from build123d import *

# Parameters (mm, degrees)
F1_DEPTH = 13.081
F2_R     = 2.54
F3_DEPTH = 25.4
F4_R     = 3.4925
F5_DEPTH = 25.4
F6_SIZE2 = 1.4664696837
F6_SIZE  = 2.54
F7_R     = 5.08


with BuildPart() as f1:
    # F0 (on Top) → F1 (new body)
    with BuildSketch(Plane.XY):
        with BuildLine():
            ThreePointArc((3.1717183454, 34.7806818182), (21.0354315126, 27.8794950829), (32.574512842, 12.5959016393))
            ThreePointArc((32.574512842, 12.5959016393), (33.9739390049, 10.8274361777), (36.1280960611, 10.16))
            Line((36.1280960611, 10.16), (40.005, 10.16))
            ThreePointArc((40.005, 10.16), (41.8010512242, 9.4160512242), (42.545, 7.62))
            Line((42.545, 7.62), (42.545, -7.62))
            Line((42.545, -7.62), (55.245, -7.62))
            Line((55.245, -7.62), (55.245, 5.1702561211))
            ThreePointArc((55.245, 5.1702561211), (54.9549810189, 6.6282799984), (54.1290768363, 7.8643329574))
            Line((54.1290768363, 7.8643329574), (21.8343329574, 40.1590768363))
            ThreePointArc((21.8343329574, 40.1590768363), (20.5982799984, 40.9849810189), (19.1402561211, 41.275))
            Line((19.1402561211, 41.275), (0, 41.275))
            Line((0, 41.275), (-56.515, 41.275))
            Line((-56.515, 41.275), (-56.515, 18.415))
            Line((-56.515, 18.415), (-43.815, 18.415))
            ThreePointArc((-43.815, 18.415), (-42.0189487758, 17.6710512242), (-41.275, 15.875))
            Line((-41.275, 15.875), (-41.275, 0))
            ThreePointArc((-41.275, 0), (-40.8262821798, -6.0696217652), (-39.4898851183, -12.0072727273))
            ThreePointArc((-39.4898851183, -12.0072727273), (-37.9470586927, -13.8847124809), (-35.528565284, -14.1213198343))
            ThreePointArc((-35.528565284, -14.1213198343), (-34.7738270947, -13.7787585984), (-34.1334673575, -13.252529236))
            ThreePointArc((-34.1334673575, -13.252529236), (-33.3596724116, -11.8025855442), (-33.414518177, -10.16))
            ThreePointArc((-33.414518177, -10.16), (-33.8417993799, -8.6306569699), (-34.1991233561, -7.0834727836))
            ThreePointArc((-34.1991233561, -7.0834727836), (-33.8811086179, 8.4750282492), (-26.836399518, 22.3509124179))
            ThreePointArc((-26.836399518, 22.3509124179), (-24.6957043329, 24.6957043329), (-22.3509124179, 26.836399518))
            ThreePointArc((-22.3509124179, 26.836399518), (-13.3652188754, 32.266492673), (-3.1717183454, 34.7806818182))
            ThreePointArc((-3.1717183454, 34.7806818182), (0, 34.925), (3.1717183454, 34.7806818182))
        make_face()
        with BuildLine():
            ThreePointArc((-26.836399518, 22.3509124179), (-22.4506403027, 22.4506403027), (-22.3509124179, 26.836399518))
            ThreePointArc((-22.3509124179, 26.836399518), (-24.6957043329, 24.6957043329), (-26.836399518, 22.3509124179))
        make_face()
        with BuildLine():
            ThreePointArc((-32.3537599551, -13.1525602742), (-30.3768347063, -9.2363636364), (-34.1991233561, -7.0834727836))
            ThreePointArc((-34.1991233561, -7.0834727836), (-33.8417993799, -8.6306569699), (-33.414518177, -10.16))
            ThreePointArc((-33.414518177, -10.16), (-32.9181630162, -11.6683404405), (-32.3537599551, -13.1525602742))
        make_face()
        with BuildLine():
            ThreePointArc((-32.3537599551, -13.1525602742), (-32.9181630162, -11.6683404405), (-33.414518177, -10.16))
            ThreePointArc((-33.414518177, -10.16), (-33.3596724116, -11.8025855442), (-34.1334673575, -13.252529236))
            ThreePointArc((-34.1334673575, -13.252529236), (-33.3085642944, -13.333231598), (-32.4908818133, -13.1976834706))
            ThreePointArc((-32.4908818133, -13.1976834706), (-32.422064403, -13.175901276), (-32.3537599551, -13.1525602742))
        make_face()
        with BuildLine():
            ThreePointArc((-32.4908818133, -13.1976834706), (-33.3085642944, -13.333231598), (-34.1334673575, -13.252529236))
            ThreePointArc((-34.1334673575, -13.252529236), (-34.7738270947, -13.7787585984), (-35.528565284, -14.1213198343))
            Line((-35.528565284, -14.1213198343), (-32.4908818133, -13.1976834706))
        make_face()
        with BuildLine():
            ThreePointArc((-3.1717183454, 34.7806818182), (0, 31.75), (3.1717183454, 34.7806818182))
            ThreePointArc((3.1717183454, 34.7806818182), (0, 34.925), (-3.1717183454, 34.7806818182))
        make_face()
    extrude(amount=F1_DEPTH)

    # F2 (on face) → F3 (cut)
    with BuildSketch(Plane.YZ.offset(55.245)):
        with Locations((-1.2248719395, 6.5405)):
            Circle(F2_R)
    extrude(amount=-F3_DEPTH, mode=Mode.SUBTRACT)

    # F4 (on face) → F5 (cut)
    with BuildSketch(Plane(origin=(0, 41.275, 0), x_dir=(-1, 0, 0), z_dir=(0, 1, 0))):
        with Locations((48.895, 6.5405)):
            Circle(F4_R)
    extrude(amount=-F5_DEPTH, mode=Mode.SUBTRACT)

    # F6
    f6_edges = [f1.edges().sort_by_distance(p)[0] for p in [
        (-45.4025, 41.275, 6.5405),
        (-45.4025, 18.415, 6.5405),
    ]]
    f6_side = f1.faces().sort_by_distance((-45.4025, 29.845, 6.5405))[0]
    chamfer(f6_edges, length=F6_SIZE, length2=F6_SIZE2, reference=f6_side)

    # F7
    f7_edges = [f1.edges().sort_by_distance(p)[0] for p in [
        (-56.515, 29.845, 13.081),
        (-56.515, 29.845, 0),
        (48.895, -7.62, 13.081),
        (48.895, -7.62, 0),
    ]]
    fillet(f7_edges, radius=F7_R)


solid = f1.part
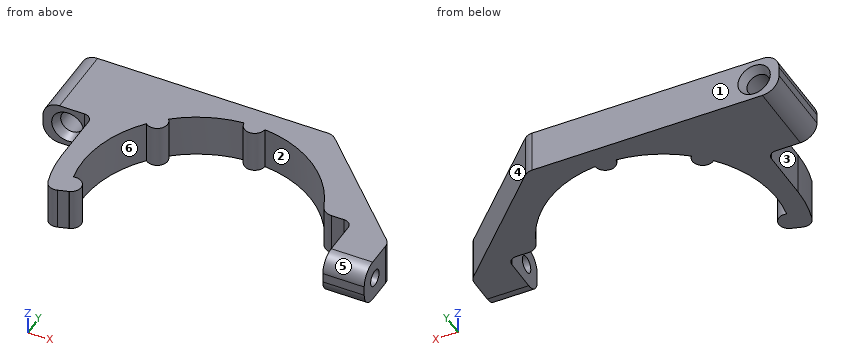
Design review of the part built by this model. Coordinates are the model's own, in mm. Face numbers are marked on the shaded views. A direction names the side the tool comes from. Coordinates: 2 decimals unless noted, no trailing zeros. Order: outer loops, then holes, each group sorted by start corner. A loop starts at its lowest first (then second) coordinate and runs counter-clockwise, first axis right, second up.
Item 1: Take a section at A-A, the plane y = 24. Write out the cut boundary in (x, z) (1 decimal).
Item 2: Take a section at B-B, the plane y = 17. Write out the cut boundary in (x, z).
Item 3: Take a section at D-D, the plane y = -10.16. Write out the cut boundary in (x, z) (3 decimals), then the cut area to 3 significant figures.
Item 4: For line 1 (Y direction, x = 48.5, z = 8.75); line 2 (X direction, y = 28, z = 8) (3 decimals); line 3 (Y direction, x = -30.5, z = 8.25) (3 decimals), list the stretches that pass through material, from the lowest coordinate up.
Item 5: The part is to be moulded in two halves that separate along X. For the marked faces 4, 5 and 6, say which applies: pulls with the +X half, pulls with the -X half, needs draft (parallel to the pull), parting line crosses it, or undercut.
Item 6: For pin 1 Ø2 at (y, z) = (6.5, 3) entering from -X (3 decimals); pin 2 Ø4.5 at (y, z) = (-1.22, 6.54) entering from +X; pin 3 Ø6.5 at (x, z) = (-48.9, 6.54) entering from +Y; pin 4 Ø2 at (x, z) = (38.5, 8) entering from +Y, all flat-tipped, find the tip position at first contact; note any pin that passes through.
Item 7: For the marked faces 1, 2 and 3, list the 3-axis set-ups (+Z, -Z, +X, -X, +Y, -Y) from which the entire face can be reached by the end or side of a thin tool; tool diameter is ignored.
Item 8: Take a section at C-C, the plane x = -19. Write out the cut boundary in (y, z) (3 decimals).
The answers:
1. outline: (-56.5, 5.1) arc R5.1 ccw to (-51.4, 0) - (-21.6, 0) - (-21.6, 13.1) - (-51.4, 13.1) arc R5.1 ccw to (-56.5, 8) - close; (25.4, 0) - (38, 0) - (38, 13.1) - (25.4, 13.1) - close; hole circle Ø7 at (-48.9, 6.5)
2. outline: (-41.54, 0) - (-30.51, 0) - (-30.51, 13.08) - (-41.54, 13.08) - close; (30.51, 0) - (44.99, 0) - (44.99, 13.08) - (30.51, 13.08) - close
3. outline: (-40.005, 0) - (-30.24, 0) - (-30.24, 13.081) - (-40.005, 13.081) - close
3. area: 128 mm2
4. line 1: y = -7.56 to -2.48, 0.03 to 13.49
4. line 2: x = -56.515 to -52.068, -45.722 to -20.875, 20.875 to 33.993
4. line 3: y = -11.419 to -8.901, 17.015 to 41.275
5. face 4: pulls with the +X half
5. face 5: needs draft
5. face 6: undercut
6. pin 1: stops at x = -41.275
6. pin 2: stops at x = -34.75
6. pin 3: passes through
6. pin 4: stops at y = 24.49
7. face 1: +Z, -Z, +X, -X, +Y
7. face 2: +Z, -Z, -Y
7. face 3: +Z, -Z, -X, -Y
8. outline: (29.305, 0) - (41.275, 0) - (41.275, 13.081) - (29.305, 13.081) - close
